Could you check a few things on this model? Use its own coordinates, in mm. A direction names the side the tool comes from. Give positions to 0.01 mm unless a question says otherwise; leave off trailing zeros. Write each loop counter-clockwise with the first axis right and the second up, starting at its lowest first coordinate (ties: lowest second). Pieces come first, ordered by that corner, then holes. Notation, with made-up numbers: (85.25, 0.25) -> (132.25, 0.25) arc R27 ccw to (132.25, 27.25) -> close; hole circle Ø10 at (-37.5, 36). An arc over 180 degrees is marked (long way). One line per question, with ' | ' between items.
from build123d import *

# Parameters (mm, degrees)
SKETCH1_W               = 50
SKETCH1_H               = 70
BOSS_EXTRUDE1_DEPTH     = 270
SHELL1_T                = -5
CUT_EXTRUDE1_DEPTH      = 277.812210713
CUT_EXTRUDE1_DEPTH_BACK = 277.812210713
SKETCH2_W               = 5
SKETCH2_H               = 60


with BuildPart() as part:
    # Sketch1 → Boss-Extrude1 (new, symmetric)
    with BuildSketch(Plane(origin=(0, 0, 0), x_dir=(-1, 0, 0), z_dir=(0, 1, 0))):
        Rectangle(SKETCH1_W, SKETCH1_H)
    extrude(amount=BOSS_EXTRUDE1_DEPTH, both=True)

    # Shell1
    shell1_openings = [part.faces().sort_by_distance(p)[0] for p in [
        (0, 270, 0),
        (0, -270, 0),
    ]]
    offset(amount=SHELL1_T, openings=shell1_openings, kind=Kind.INTERSECTION)

    # Sketch2 → Cut-Extrude1 (cut, two sides: drawn at the far end of the back side and taken through both)
    with BuildSketch(Plane.YZ.offset(25).offset(-CUT_EXTRUDE1_DEPTH_BACK)):
        with Locations((-262.5, 0)):
            Rectangle(SKETCH2_W, SKETCH2_H)
        with Locations((-207.5, 0)):
            Rectangle(SKETCH2_W, SKETCH2_H)
        with Locations((207.5, 0)):
            Rectangle(SKETCH2_W, SKETCH2_H)
        with Locations((262.5, 0)):
            Rectangle(SKETCH2_W, SKETCH2_H)
    extrude(amount=CUT_EXTRUDE1_DEPTH + CUT_EXTRUDE1_DEPTH_BACK, mode=Mode.SUBTRACT)


solid = part.part
Q1. Imagine slicing it at B-B on y = -45. Please give me the cut outline in (x, z), and give its area (3 significant figures).
Answer below:
outline: (-25, -35) -> (25, -35) -> (25, 35) -> (-25, 35) -> close; hole (-20, -30) -> (20, -30) -> (20, 30) -> (-20, 30) -> close | area: 1,100 mm^2
Q2. Imagine slicing it at A-A on x = 11. Please give me the cut outline in (y, z).
Answer below:
outline: (-270, -35) -> (270, -35) -> (270, -30) -> (-270, -30) -> close; (-270, 30) -> (270, 30) -> (270, 35) -> (-270, 35) -> close
Q3. On a 3-axis mill with a long thin cutter (end or side, diameter ignored), from which of +Z, -Z, +X, -X, +Y, -Y can I reach the whole of each face in a straight line? I mean faces 1 (the flat face through (0, 4, -35)), 2 (the flat face through (-20, -235, 0)). Say none if no direction works.
Answer below:
face 1: -Z, +X, -X, +Y, -Y | face 2: +Y, -Y
Q4. If I drill on line 1 along X through (y, z) = (146, 24); line 2 along Z through (x, y) = (-18, 96); line 3 along Y through (x, z) = (20.5, 22), over which ranges is the centre line in solid material (lowest first)?
Answer below:
line 1: x = -25 to -20, 20 to 25 | line 2: z = -35 to -30, 30 to 35 | line 3: y = -270 to -265, -260 to -210, -205 to 205, 210 to 260, 265 to 270
Q5. If we mould it in two halves opening along Z, with no side actions, what happens to faces 3 (the flat face through (-20, 3, 0)), 4 (the flat face through (23, -270, 0)), 5 (the flat face through (0, 4, 35))? For each: +Z half, -Z half, draft (parallel to the pull), parting line (faces both ways), or undercut.
Answer below:
face 3: undercut | face 4: draft | face 5: +Z half
Q6. Imagine slicing it at C-C on z = -13.5. Count the separate pieces of the cut face and the enclosed holes in it, and give its area (3 significant figures).
Answer below:
separate pieces: 10 | enclosed holes: 0 | area: 5,200 mm^2
